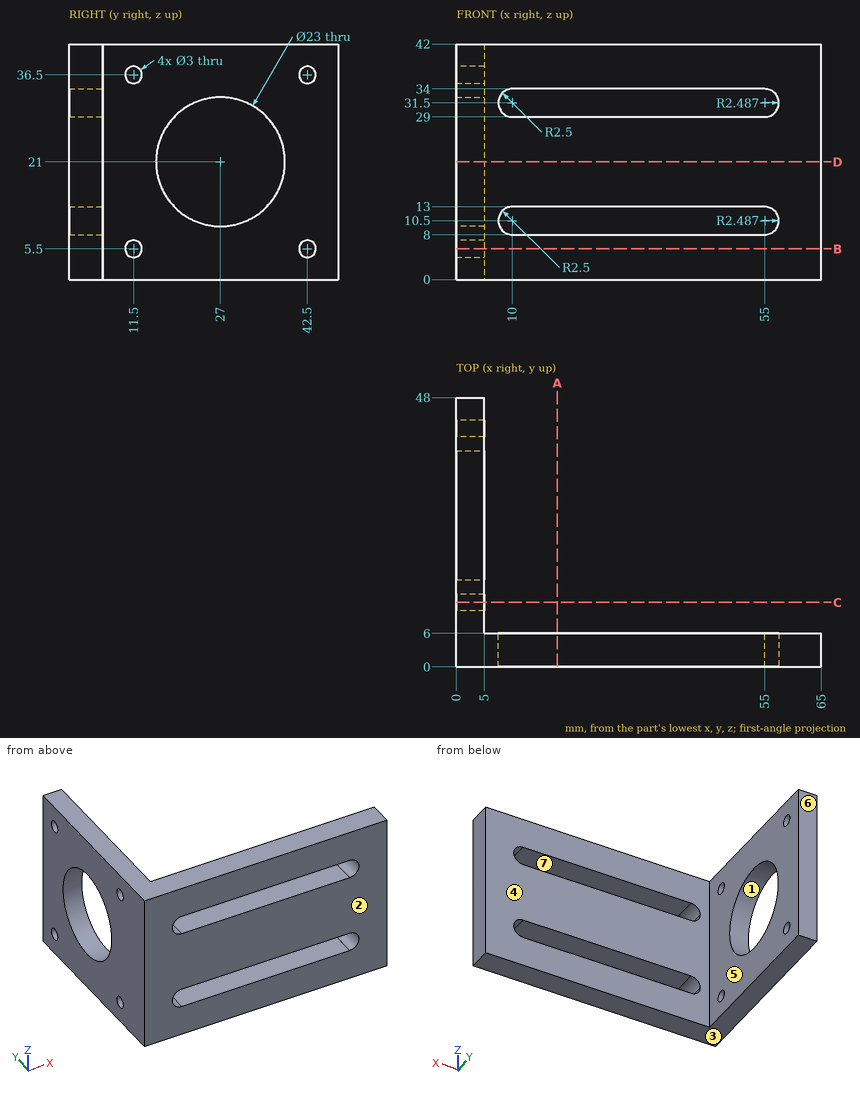
The figure shows three views and two pictorial views of one solid part (mm, origin at its lowest corner). Answer the questions. A direction names the side the tool comes from. Give positions to 0.01 mm unless a question says otherwise; leave off trailing zeros. Loops run counter-clockwise (first coordinate to the right, second up) from the corner with the lowest first, then second, coordinate; pieces in that order, holes last. Notation, with made-up numbers: (63.25, 15) -> (77.25, 15) arc R38 ccw to (77.25, 54) -> close; hole circle Ø2 at (-28, 1.5). An arc over 180 degrees is marked (long way). Use a Markdown table: item, result. Add a question column.
1. Section C-C on y = 11.5 is taken. Determine the outline of the cut face in (x, z).
2. For the marked faces 5, 6 and 7, determine the directions among +Z, -Z, +X, -X, +Y, -Y from which every point of the face is accessible in a straight line to the end or side of a thin tool.
3. Section D-D on z = 21 is taken. Determine the outline of the cut face in (x, y).
4. Find the intervals of material crossed by probe 1 along Z at (x, y) = (31, 4.5); probe 2 along Y at (x, z) = (1.95, 5.5); probe 3 along Y at (x, z) = (2, 36), in increasing order.
5. Section A-A on x = 18 is taken. Determine the outline of the cut face in (y, z).
6. Flat-ended cylindrical pins translate along their axes: pin 1 Ø3.5 at (y, z) = (11.5, 5.5) entering from +X; pin 2 Ø12 at (x, z) = (28, 24) entering from +Y. Find the tip coordinate at first contact, or state that the pin passes through.
7. Determine the mould class of the marked faces 1, 2, 3 and 4 for opening direction Y: released by +Y, released by -Y, zero draft, split by the parting line, or undercut.
8. Section B-B on z = 5.5 is taken. Determine the outline of the cut face in (x, y), and give its area (3 significant figures).
Results below:
| question | item | result |
|---|---|---|
| 1 | outline | (0, 0) -> (5, 0) -> (5, 4) -> (0, 4) -> close; (0, 7) -> (5, 7) -> (5, 35) -> (0, 35) -> close; (0, 38) -> (5, 38) -> (5, 42) -> (0, 42) -> close |
| 2 | face 5 | +Z, -Z, +X, +Y |
| 2 | face 6 | +Z, -Z, +X, -X, +Y |
| 2 | face 7 | +Y, -Y |
| 3 | outline | (0, 0) -> (65, 0) -> (65, 6) -> (5, 6) -> (5, 15.5) -> (0, 15.5) -> close; (0, 38.5) -> (5, 38.5) -> (5, 48) -> (0, 48) -> close |
| 4 | probe 1 | z = 0 to 8, 13 to 29, 34 to 42 |
| 4 | probe 2 | y = 0 to 10, 13 to 41, 44 to 48 |
| 4 | probe 3 | y = 0 to 10.09, 12.91 to 41.09, 43.91 to 48 |
| 5 | outline | (0, 0) -> (6, 0) -> (6, 8) -> (0, 8) -> close; (0, 13) -> (6, 13) -> (6, 29) -> (0, 29) -> close; (0, 34) -> (6, 34) -> (6, 42) -> (0, 42) -> close |
| 6 | pin 1 | stops at x = 5 |
| 6 | pin 2 | stops at y = 6 |
| 7 | face 1 | undercut |
| 7 | face 2 | released by -Y |
| 7 | face 3 | zero draft |
| 7 | face 4 | released by +Y |
| 8 | outline | (0, 0) -> (65, 0) -> (65, 6) -> (5, 6) -> (5, 10) -> (0, 10) -> close; (0, 13) -> (5, 13) -> (5, 41) -> (0, 41) -> close; (0, 44) -> (5, 44) -> (5, 48) -> (0, 48) -> close |
| 8 | area | 570 mm^2 |
